Here's how the part is built. I have some questions about the finished solid (model axes, mm). A direction names the side the tool comes from. Coordinates: 2 decimals unless noted, no trailing zeros. Order: outer loops, then holes, each group sorted by start corner. A loop starts at its lowest first (then second) coordinate and runs counter-clockwise, first axis right, second up. Notation, with made-up numbers: (-8.5, 19.25) - (37.5, 19.25) arc R29 cw to (37.5, 40.25) - close; hole circle Ø9 at (-15, 85). An arc over 180 degrees is marked (long way). Answer in a Markdown table with one row per item. Add a question column.
Item 1: I want a section at D-D (x = 81.75). Please give me the cut outline in (y, z), plus the area to 3 significant figures.
Item 2: Will these pins go through, and if not, where does the flat tip stop? pin 1 Ø3 at (y, z) = (11.5, -9.5) entering from +X; pin 2 Ø2 at (y, z) = (12, -10) entering from -X; pin 3 Ø3 at (x, y) = (82.5, 14.5) entering from -Z.
Item 3: If I drill on line 1 along Y through (x, z) = (92.75, -10); line 2 along Y through (x, z) = (94.25, 0); line 3 along Z through (x, y) = (89, 12), over which ranges is the centre line in solid material (lowest first)? Write a range as from..to.
Item 4: I want a section at A-A (z = 0). Please give me the cut outline in (x, y).
Item 5: I want a section at C-C (y = 8.5). Please give me the cut outline in (x, z) (3 decimals).
Item 6: Thinking about a two-plate mould opening in Y: for faces 1 (the cylindrical face through (78, 9, 0)), 2 (the flat face through (80, 9, 0)), 3 (the flat face through (88, 17, 0)), 4 (the flat face through (80, 12, -10)), which applies, +Y half, -Y half, draft (parallel to the pull), parting line (faces both ways), or undercut?
Item 7: I want a section at B-B (x = 95). Please give me the cut outline in (y, z).
Item 8: On a 3-axis mill with a long thin cutter (end or side, diameter ignored), from which of +Z, -Z, +X, -X, +Y, -Y can I reach the whole of each face in a straight line? I mean faces 5 (the flat face through (86.525, 8.619, -15.257)), 6 (the cylindrical face through (88.685, 13.138, 9.274)). Say none if no direction works.
```python
from build123d import *

# Parameters (mm, degrees)
SKETCH1_W          = 20
SKETCH1_H          = 17
REVOLVE1_ANGLE     = 20
SKETCH2_R          = 2.5
SKETCH2_R_2        = 1.35
CUT_EXTRUDE1_DEPTH = 20


with BuildPart() as part:
    # Sketch1 → Revolve1 (revolve, symmetric)
    with BuildSketch(Plane.XY) as revolve1_sk:
        with Locations((88, 8.5)):
            Rectangle(SKETCH1_W, SKETCH1_H)
    revolve(axis=Axis((0, -55, 0), (0, 1, 0)), revolution_arc=REVOLVE1_ANGLE / 2)
    revolve(revolve1_sk.sketch, axis=Axis((0, -55, 0), (0, -1, 0)), revolution_arc=REVOLVE1_ANGLE / 2)

    # Sketch2 → Cut-Extrude1 (cut)
    with BuildSketch(Plane(origin=(80, 0, 0), x_dir=(0, 0, -1), z_dir=(1, 0, 0))):
        with Locations((0, 8.5)):
            Circle(SKETCH2_R)
        with Locations((-10, 12)):
            Circle(SKETCH2_R_2)
        with Locations((10, 12)):
            Circle(SKETCH2_R_2)
    extrude(amount=CUT_EXTRUDE1_DEPTH, mode=Mode.SUBTRACT)


solid = part.part
```
Values follow:
| question | item | result |
|---|---|---|
| 1 | outline | (0, -14.41) - (17, -14.41) - (17, 14.41) - (0, 14.41) - close; hole circle Ø5 at (8.5, 0); hole circle Ø2.7 at (12, -10); hole circle Ø2.7 at (12, 10) |
| 1 | area | 459 mm^2 |
| 2 | pin 1 | stops at x = 97.67 |
| 2 | pin 2 | stops at x = 77.22 |
| 2 | pin 3 | stops at z = -14.81 |
| 3 | line 1 | y = 0..10.65, 13.35..17 |
| 3 | line 2 | y = 0..6, 11..17 |
| 3 | line 3 | z = -15.69..-11.35, -8.65..8.65, 11.35..15.69 |
| 4 | outline | (78, 0) - (98, 0) - (98, 6) - (80, 6) - (80, 11) - (98, 11) - (98, 17) - (78, 17) - close |
| 5 | outline | (76.815, -13.545) - (96.511, -17.018) arc R98 ccw to (97.968, -2.5) - (80, -2.5) - (80, 2.5) - (97.968, 2.5) arc R98 ccw to (96.511, 17.018) - (76.815, 13.545) arc R78 cw to start |
| 6 | face 1 | draft |
| 6 | face 2 | undercut |
| 6 | face 3 | +Y half |
| 6 | face 4 | undercut |
| 7 | outline | (0, -16.75) - (17, -16.75) - (17, 16.75) - (0, 16.75) - close; hole circle Ø5 at (8.5, 0); hole circle Ø2.7 at (12, -10); hole circle Ø2.7 at (12, 10) |
| 8 | face 5 | -Z, -X, +Y, -Y |
| 8 | face 6 | +X |
